```python
from build123d import *

# Parameters (mm, degrees)
SKETCH2_W               = 50.8
SKETCH2_H               = 25.4
SKETCH2_W_2             = 47.625
SKETCH2_H_2             = 22.225
BOSS_EXTRUDE1_DEPTH     = 152.4
SKETCH3_R               = 14.2875
CUT_EXTRUDE1_DEPTH      = 157.576115675
CUT_EXTRUDE2_DEPTH      = 162.144934764
CUT_EXTRUDE2_DEPTH_BACK = 162.144934764
SKETCH4_R               = 2.54


with BuildPart() as part:
    # Sketch2 → Boss-Extrude1 (new, symmetric)
    with BuildSketch(Plane.XY):
        Rectangle(SKETCH2_W, SKETCH2_H)
        Rectangle(SKETCH2_W_2, SKETCH2_H_2, mode=Mode.SUBTRACT)
    extrude(amount=BOSS_EXTRUDE1_DEPTH, both=True)

    # Sketch3 → Cut-Extrude1 (cut, through all)
    with BuildSketch(Plane(origin=(0, 12.7, 0), x_dir=(1, 0, 0), z_dir=(0, 1, 0))):
        with Locations(Location((0, -88.9, 0), (0, 0, 270))):
            Circle(SKETCH3_R)
        with Locations(Location((0, -22.225, 0), (0, 0, 270))):
            Circle(SKETCH3_R)
        with Locations(Location((0, 22.225, 0), (0, 0, 90))):
            Circle(SKETCH3_R)
        with Locations(Location((0, 88.9, 0), (0, 0, 90))):
            Circle(SKETCH3_R)
    extrude(amount=-CUT_EXTRUDE1_DEPTH, mode=Mode.SUBTRACT)

    # Sketch4 → Cut-Extrude2 (cut, two sides: drawn at the far end of the back side and taken through both)
    with BuildSketch(Plane.ZY.offset(25.4).offset(-CUT_EXTRUDE2_DEPTH_BACK)):
        with Locations((-142.875, 6.35)):
            Circle(SKETCH4_R)
        with Locations((-142.875, -6.35)):
            Circle(SKETCH4_R)
        with Locations((-117.475, 6.35)):
            Circle(SKETCH4_R)
        with Locations((-117.475, -6.35)):
            Circle(SKETCH4_R)
        with Locations((117.475, -6.35)):
            Circle(SKETCH4_R)
        with Locations((117.475, 6.35)):
            Circle(SKETCH4_R)
        with Locations((142.875, -6.35)):
            Circle(SKETCH4_R)
        with Locations((142.875, 6.35)):
            Circle(SKETCH4_R)
    extrude(amount=CUT_EXTRUDE2_DEPTH + CUT_EXTRUDE2_DEPTH_BACK, mode=Mode.SUBTRACT)


solid = part.part
```
CAD build for the part. Positions are in the model's coordinates, mm. A direction names the side the tool comes from. Give positions to 0.01 mm unless a question says otherwise; leave off trailing zeros. Order: outer loops, then holes, each group sorted by start corner. A loop starts at its lowest first (then second) coordinate and runs counter-clockwise, first axis right, second up.
(1) Saw through at D-D, the plane z = -33.5. Give the cut face in (x, y), then the cut area to 3 significant figures.
(2) Drill centre lines: L1, parallel to Z at x = 24.3, y = 6.35 (3 decimals); L2, parallel to X at y = -3.5, z = 79; L3, parallel to Y at x = -7.5, z = 45. Where is each one in solid material? Low to high.
(3) Saw through at C-C, the plane y = -6.35. State how many separate pieces and enclosed holes the cut face has, then the cut area to 3 significant figures.
(4) Tool access for faces 4 (the flat face through (23.812, 0, 2)), 5 (the cylindrical face through (-0.63, 11.92, -7.95)): list every direction of +Z, -Z, +X, -X, +Y, -Y with a clear straight run to the whole face (end or side of a thin tool).
(5) Saw through at B-B, the plane x = 19.5. Give the cut face in (y, z), then the cut area to 3 significant figures.
(6) Flat gauge pin, fed straight in: pin 1 (23 mm diameter, centred on x = 0, z = -22.225, fed in from +Y). Where does the tip first touch, or does it go through?
(7) Mould opens along Y. For faces 1 (the cylindrical face through (24.6, 7.1, 119.9)), 2 (the flat face through (0, -12.7, 2)), 3 (the flat face through (0, -12, -152.4)) say: released by +Y, released by -Y, zero draft, split by the parting line, or undercut.
(8) Saw through at A-A, the plane z = -88.9. Give the cut face in (x, y), then the cut area to 3 significant figures.
Results found:
1. outline: (-25.4, -12.7) - (-8.78, -12.7) - (-8.78, -11.11) - (-23.81, -11.11) - (-23.81, 11.11) - (-8.78, 11.11) - (-8.78, 12.7) - (-25.4, 12.7) - close; (8.78, -12.7) - (25.4, -12.7) - (25.4, 12.7) - (8.78, 12.7) - (8.78, 11.11) - (23.81, 11.11) - (23.81, -11.11) - (8.78, -11.11) - close
1. area: 176 mm2
2. L1: z = -152.4 to -145.415, -140.335 to -120.015, -114.935 to 114.935, 120.015 to 140.335, 145.415 to 152.4
2. L2: x = -25.4 to -23.81, 23.81 to 25.4
2. L3: y = -12.7 to -11.11, 11.11 to 12.7
3. separate pieces: 10
3. enclosed holes: 0
3. area: 903 mm2
4. face 4: +Z, -Z
4. face 5: +Y, -Y
5. outline: (-12.7, -152.4) - (-11.11, -152.4) - (-11.11, 152.4) - (-12.7, 152.4) - close; (11.11, -152.4) - (12.7, -152.4) - (12.7, 152.4) - (11.11, 152.4) - close
5. area: 968 mm2
6. pin 1: passes through
7. face 1: undercut
7. face 2: released by -Y
7. face 3: zero draft
8. outline: (-25.4, -12.7) - (-14.29, -12.7) - (-14.29, -11.11) - (-23.81, -11.11) - (-23.81, 11.11) - (-14.29, 11.11) - (-14.29, 12.7) - (-25.4, 12.7) - close; (14.29, -12.7) - (25.4, -12.7) - (25.4, 12.7) - (14.29, 12.7) - (14.29, 11.11) - (23.81, 11.11) - (23.81, -11.11) - (14.29, -11.11) - close
8. area: 141 mm2
